```python
from build123d import *

# Parameters (mm, degrees)
IZIM1_W                          = 8
IZIM1_H                          = 8
Y_KSEKLIK_EKSTR_ZYON1_DEPTH      = 3
KES_EKSTR_ZYON1_DEPTH            = 2
Y_KSEKLIK_EKSTR_ZYON2_DEPTH      = 7
Y_KSEKLIK_EKSTR_ZYON2_DEPTH_BACK = 3
IZIM3_W                          = 2
IZIM3_H                          = 8
IZIM4_W                          = 7
IZIM4_H                          = 2
Y_KSEKLIK_EKSTR_ZYON3_DEPTH      = 8
IZIM5_R                          = 1.5
KES_EKSTR_ZYON2_DEPTH            = 7
IZIM7_R                          = 1.5
KES_EKSTR_ZYON3_DEPTH            = 7


with BuildPart() as part:
    # Çizim1 → Yükseklik-Ekstrüzyon1 (new body)
    with BuildSketch(Plane.XY):
        with Locations((4, 4)):
            Rectangle(IZIM1_W, IZIM1_H)
    extrude(amount=Y_KSEKLIK_EKSTR_ZYON1_DEPTH)

    # Çizim2 → Kes-Ekstrüzyon1 (cut)
    with BuildSketch(Plane.XY.offset(3)):
        Polygon((5.58771324, 6.75), (2.41228676, 6.75), (0.824573519, 4), (2.41228676, 1.25), (5.58771324, 1.25), (7.175426481, 4), align=None)
    extrude(amount=-KES_EKSTR_ZYON1_DEPTH, mode=Mode.SUBTRACT)

    # Çizim3 → Yükseklik-Ekstrüzyon2 (add, two sides: drawn at the far end of the back side and taken through both)
    with BuildSketch(Plane.XY.offset(3).offset(-Y_KSEKLIK_EKSTR_ZYON2_DEPTH_BACK)):
        with Locations((-1, 4)):
            Rectangle(IZIM3_W, IZIM3_H)
        with Locations((9, 4)):
            Rectangle(IZIM3_W, IZIM3_H)
    extrude(amount=Y_KSEKLIK_EKSTR_ZYON2_DEPTH + Y_KSEKLIK_EKSTR_ZYON2_DEPTH_BACK)

    # Çizim4 → Yükseklik-Ekstrüzyon3 (add)
    with BuildSketch(Plane(origin=(0, 8, 0), x_dir=(1, 0, 0), z_dir=(0, 1, 0))):
        with Locations((-5.5, -9)):
            Rectangle(IZIM4_W, IZIM4_H)
        with Locations((13.5, -9)):
            Rectangle(IZIM4_W, IZIM4_H)
    extrude(amount=-Y_KSEKLIK_EKSTR_ZYON3_DEPTH)

    # Çizim5 → Kes-Ekstrüzyon2 (cut)
    with BuildSketch(Plane.XY.offset(1)):
        with Locations((4, 4)):
            Circle(IZIM5_R)
    extrude(amount=-KES_EKSTR_ZYON2_DEPTH, mode=Mode.SUBTRACT)

    # Çizim7 → Kes-Ekstrüzyon3 (cut)
    with BuildSketch(Plane(origin=(0, 0, 8), x_dir=(-1, 0, 0), z_dir=(0, 0, -1))):
        with Locations((-13.5, 4)):
            Circle(IZIM7_R)
        with Locations((5.5, 4)):
            Circle(IZIM7_R)
    extrude(amount=-KES_EKSTR_ZYON3_DEPTH, mode=Mode.SUBTRACT)


solid = part.part
```
Check sheet for the modelled part. Datum: model origin and axes. Units: mm. A direction names the side the tool comes from. Round coordinates to 2 decimals unless told otherwise and drop trailing zeros. Order: outer loops, then holes, each group sorted by start corner. A loop starts at its lowest first (then second) coordinate and runs counter-clockwise, first axis right, second up. Notation, with made-up numbers: M -12.75,46.5 L 40.25,46.5 A19 cw 40.25,66.5 Z; hole C 10,77 d2. An arc over 180 degrees is marked long. Answer in a Markdown table with one row per item.
(1) Set-up check for faces 3 (the flat face through (8, 4, 6)), 4 (the flat face through (6.37, 2.606, 2.014)), 5 (the flat face through (-6, 2, 8)), 6 (the flat face through (11, 4, 10)), 7 (the flat face through (10, 4, 4)): record each of +Z, -Z, +X, -X, +Y, -Y from which the full face is reachable in a straight line by a thin tool's end or side.
Findings:
| item | result |
|---|---|
| face 3 | +Z, +Y, -Y |
| face 4 | +Z |
| face 5 | -Z, -X, +Y, -Y |
| face 6 | +Z, +X, -X, +Y, -Y |
| face 7 | -Z, +X, +Y, -Y |
(2) Draft check along Y on faces 1 (the flat face through (0, 4, 6)), 2 (the flat face through (1.61, 2.64, 2.01)). Enter one of: +Y half, -Y half, draft (parallel to the pull), parting line (faces both ways), or undercut.
Findings:
| item | result |
|---|---|
| face 1 | draft |
| face 2 | undercut |
(3) Section check B-B on x = 13.5. Record the boundary of the cut face in (y, z).
Findings:
| item | result |
|---|---|
| outline | M 0,8 L 2.5,8 L 2.5,10 L 0,10 Z; M 5.5,8 L 8,8 L 8,10 L 5.5,10 Z |
(4) Material ranges on line 1 along X through (y, z) = (6.75, 9.75); line 2 along X through (y, z) = (2.25, 6.5); line 3 along X through (y, z) = (3.25, 9), recorded low to high. Write a range as from..to.
Findings:
| item | result |
|---|---|
| line 1 | x = -9..0, 8..17 |
| line 2 | x = -2..0, 8..10 |
| line 3 | x = -9..-6.8, -4.2..0, 8..12.2, 14.8..17 |
(5) Section check C-C on z = 0.5. Record the boundary of the cut face in (x, y), plus the area to 3 significant figures.
Findings:
| item | result |
|---|---|
| outline | M -2,0 L 10,0 L 10,8 L -2,8 Z; hole C 4,4 d3 |
| area | 88.9 mm^2 |
(6) Gauge pin test, flat ends, axial feed: pin 1 (3.5 mm diameter, centred on y = 4, z = 5, fed in from -X); pin 2 (2.5 mm diameter, centred on x = 4, y = 4, fed in from -Z); pin 3 (3.5 mm diameter, centred on x = -5.5, y = 4, fed in from -Z). Record the tip position at first contact, or that the pin passes through.
Findings:
| item | result |
|---|---|
| pin 1 | stops at x = -2 |
| pin 2 | passes through |
| pin 3 | stops at z = 8 |
(7) Section check D-D on y = 0.5. Record the boundary of the cut face in (x, z).
Findings:
| item | result |
|---|---|
| outline | M -9,8 L -2,8 L -2,0 L 10,0 L 10,8 L 17,8 L 17,10 L 8,10 L 8,3 L 0,3 L 0,10 L -9,10 Z |
(8) Section check A-A on z = 5. Record the boundary of the cut face in (x, y).
Findings:
| item | result |
|---|---|
| outline | M -2,0 L 0,0 L 0,8 L -2,8 Z; M 8,0 L 10,0 L 10,8 L 8,8 Z |
